Build history of the part. All positions in model axes, mm. A direction names the side the tool comes from. Round coordinates to 2 decimals unless told otherwise and drop trailing zeros. Order: outer loops, then holes, each group sorted by start corner. A loop starts at its lowest first (then second) coordinate and runs counter-clockwise, first axis right, second up. Notation, with made-up numbers: M -16,-15 L 20,-15 A25 cw 20,10 Z; hole C 61,9 d10. An arc over 180 degrees is marked long. Use CSV: the item, a comma, the result in double quotes.
from build123d import *

# Parameters (mm, degrees)
BOX002_W     = 4.9
BOX002_H     = 12.4
BOX002_DEPTH = 16
BOX003_W     = 4.9
BOX003_H     = 12.4
BOX003_DEPTH = 16
BOX001_W     = 4.9
BOX001_H     = 12.4
BOX001_DEPTH = 16
BOX_W        = 52
BOX_H        = 20
BOX_DEPTH    = 15


with BuildPart() as cubo002:
    # Box002 → Box002 (new body)
    with BuildSketch(Plane(origin=(43.5, 3, 0), x_dir=(1, 0, 0), z_dir=(0, 0, 1))):
        with Locations((2.45, 6.2)):
            Rectangle(BOX002_W, BOX002_H)
    extrude(amount=BOX002_DEPTH)


with BuildPart() as cubo003:
    # Box003 → Box003 (new body)
    with BuildSketch(Plane(origin=(23.5, 3, 0), x_dir=(1, 0, 0), z_dir=(0, 0, 1))):
        with Locations((2.45, 6.2)):
            Rectangle(BOX003_W, BOX003_H)
    extrude(amount=BOX003_DEPTH)


with BuildPart() as cubo001:
    # Box001 → Box001 (new body)
    with BuildSketch(Plane(origin=(3.5, 3, 0), x_dir=(1, 0, 0), z_dir=(0, 0, 1))):
        with Locations((2.45, 6.2)):
            Rectangle(BOX001_W, BOX001_H)
    extrude(amount=BOX001_DEPTH)


with BuildPart() as cut002:
    # Box → Box (new body)
    with BuildSketch(Plane.XY):
        with Locations((26, 10)):
            Rectangle(BOX_W, BOX_H)
    extrude(amount=BOX_DEPTH)

    # Cut: cut Cubo001
    add(cubo001.part, mode=Mode.SUBTRACT)

    # Cut001: cut Cubo003
    add(cubo003.part, mode=Mode.SUBTRACT)

    # Cut002: cut Cubo002
    add(cubo002.part, mode=Mode.SUBTRACT)


solid = cut002.part
(1) Drop a flat-ended pin along its axis: pin 1 (4 mm diameter, centred on y = 10, z = 4, fed in from -X). Give the stop position or say it passes through.
Answer block:
pin 1,"stops at x = 0"
(2) Wall check: line 1 (X direction, y = 11, z = 10); line 2 (Y direction, x = 5.5, z = 4). Give the ranges that are in metal, low to high. Write a range as from..to.
Answer block:
line 1,"x = 0..3.5, 8.4..23.5, 28.4..43.5, 48.4..52"
line 2,"y = 0..3, 15.4..20"
(3) Cut at B-B, the plane z = 2.5. Give the cut face in (x, y).
Answer block:
outline,"M 0,0 L 52,0 L 52,20 L 0,20 Z; hole M 3.5,3 L 8.4,3 L 8.4,15.4 L 3.5,15.4 Z; hole M 23.5,3 L 28.4,3 L 28.4,15.4 L 23.5,15.4 Z; hole M 43.5,3 L 48.4,3 L 48.4,15.4 L 43.5,15.4 Z"
(4) Cut at A-A, the plane y = 3.75. Give the cut face in (x, z), and give its area (4 significant figures).
Answer block:
outline,"M 0,0 L 3.5,0 L 3.5,15 L 0,15 Z; M 8.4,0 L 23.5,0 L 23.5,15 L 8.4,15 Z; M 28.4,0 L 43.5,0 L 43.5,15 L 28.4,15 Z; M 48.4,0 L 52,0 L 52,15 L 48.4,15 Z"
area,"559.5 mm²"
(5) Tool access for faces 4 (the face through (26, 3, 7)), 5 (the face through (26, 0, 7)): list every direction of +Z, -Z, +X, -X, +Y, -Y with a clear straight run to the whole face (end or side of a thin tool).
Answer block:
face 4,"+Z, -Z"
face 5,"+Z, -Z, +X, -X, -Y"
(6) Two-plate mould, pull along X, no slides. Class faces 1 (the face through (0, 10, 7)), 2 (the face through (31, 10, 0)), 3 (the face through (28.4, 9, 7)): released by +X, released by -X, zero draft, split by the parting line, or undercut.
Answer block:
face 1,"released by -X"
face 2,"zero draft"
face 3,"undercut"
